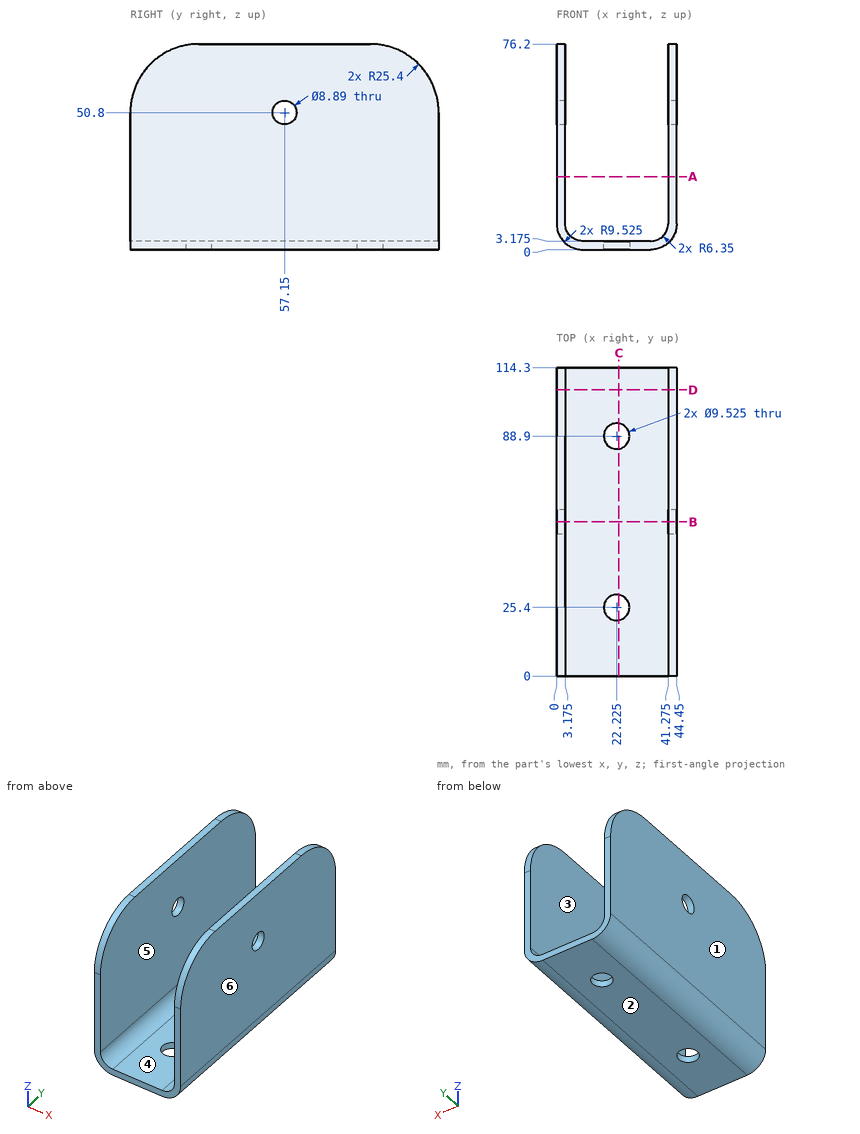
Check sheet for the drawn part. Datum: minimum x, y, z corner. Units: mm. A direction names the side the tool comes from. Round coordinates to 2 decimals unless told otherwise and drop trailing zeros. Order: outer loops, then holes, each group sorted by start corner. A loop starts at its lowest first (then second) coordinate and runs counter-clockwise, first axis right, second up.
1) Section check D-D (y = 106). Record the boundary of the cut face in (x, z) (3 decimals).
2) Scan lines: line 1 (X direction, y = 41.5, z = 49) (3 decimals); line 2 (Z direction, x = 42, y = 43); line 3 (Z direction, x = 29.5, y = 13.5) (3 decimals). Record each from-to range of solid material in increasing order.
3) Tool access check on the marked faces 5 and 6. Record the directions out of +Z, -Z, +X, -X, +Y, -Y that give a thin tool (end or side, any length) a straight path to the whole face; none if there is none.
4) Section check B-B (y = 57.15). Record the boundary of the cut face in (x, z) (3 decimals).
5) Section check A-A (z = 27). Record the boundary of the cut face in (x, y) (3 decimals).
6) Mould release check, pull along X, two halves, no side actions. Record for the marked faces 1, 2, 3 and 4: +X half, -X half, draft (parallel to the pull), parting line (faces both ways), or undercut.
7) Section check C-C (x = 23). Record the boundary of the cut face in (y, z) (3 decimals), and give its area (3 significant figures).
8) Go/stop test with flat-tipped pins: pin 1 Ø14 at (y, z) = (57.15, 50.8) entering from -X; pin 2 Ø7.5 at (x, y) = (27, 72) entering from +Z (3 decimals). Record where each tip stops, or that it passes through.
Result:
1. outline: (0, 9.525) arc R9.525 ccw to (9.525, 0) - (34.925, 0) arc R9.525 ccw to (44.45, 9.525) - (44.45, 69.582) - (41.275, 69.582) - (41.275, 9.525) arc R6.35 cw to (34.925, 3.175) - (9.525, 3.175) arc R6.35 cw to (3.175, 9.525) - (3.175, 69.582) - (0, 69.582) - close
2. line 1: x = 0 to 3.175, 41.275 to 44.45
2. line 2: z = 3.15 to 76.2
2. line 3: z = 0 to 3.175
3. face 5: +Z, +Y, -Y
3. face 6: +Z, -Z, +X, +Y, -Y
4. outline: (0, 9.525) arc R9.525 ccw to (9.525, 0) - (34.925, 0) arc R9.525 ccw to (44.45, 9.525) - (44.45, 46.355) - (41.275, 46.355) - (41.275, 9.525) arc R6.35 cw to (34.925, 3.175) - (9.525, 3.175) arc R6.35 cw to (3.175, 9.525) - (3.175, 46.355) - (0, 46.355) - close; (0, 55.245) - (3.175, 55.245) - (3.175, 76.2) - (0, 76.2) - close; (41.275, 55.245) - (44.45, 55.245) - (44.45, 76.2) - (41.275, 76.2) - close
5. outline: (0, 0) - (3.175, 0) - (3.175, 114.3) - (0, 114.3) - close; (41.275, 0) - (44.45, 0) - (44.45, 114.3) - (41.275, 114.3) - close
6. face 1: -X half
6. face 2: draft
6. face 3: undercut
6. face 4: undercut
7. outline: (0, 0) - (20.701, 0) - (20.701, 3.175) - (0, 3.175) - close; (30.099, 0) - (84.201, 0) - (84.201, 3.175) - (30.099, 3.175) - close; (93.599, 0) - (114.3, 0) - (114.3, 3.175) - (93.599, 3.175) - close
7. area: 303 mm2
8. pin 1: stops at x = 0
8. pin 2: stops at z = 3.175
